Autodesk Inventor part; units mm, degrees
ref_plane "YZ Plane" through (0, 0, 0) normal (1, 0, 0) x (0, 1, 0)
ref_plane "XZ Plane" through (0, 0, 0) normal (0, 1, 0) x (-1, 0, 0)
ref_plane "XY Plane" through (0, 0, 0) normal (0, 0, 1) x (1, 0, 0)
sketch "Sketch1" plane through (0, 0, 0) normal (0, 0, 1) x (1, 0, 0)
  circle A0 centre (0, 0) radius 5
  circle A1 centre (0, 0) radius 7
  dimension "d0" = 10
  dimension "d1" = 14
extrude "Extrusion1" add sketch "Sketch1" along normal blind 12.7
sketch "Sketch2" plane through (0, 0, 12.7) normal (0, 0, 1) x (1, 0, 0)
  circle A0 centre (0, 0) radius 7
  dimension "d14" = 14
extrude "Extrusion2" add sketch "Sketch2" along normal blind 19.25
chamfer "Chamfer1" distance 0.4128 angle 45 1 edges at (-5, 0, 0)
thread "Thread1"
sketch "Sketch3" plane through (0, 0, 31.95) normal (0, 0, 1) x (1, 0, 0)
  circle A0 centre (0, 0) radius 5
  dimension "d11" = 10
extrude "Extrusion3" add sketch "Sketch3" along normal blind 12.7
thread "Thread2"
sketch "Sketch4" plane through (0, 0, 44.65) normal (0, 0, 1) x (1, 0, 0)
  line L0 (2.54, 0.635) -> (-2.54, 0.635)
  line L1 (-2.54, 0.635) -> (-2.54, -0.635)
  line L2 (-2.54, -0.635) -> (2.54, -0.635)
  line L3 (2.54, -0.635) -> (2.54, 0.635)
  line L4 (2.54, 0.635) -> (-2.54, -0.635) construction
  line L5 (-2.54, 0.635) -> (2.54, -0.635) construction
  point P0 (0, 0)
  dimension "d17" = 5.08
  dimension "d18" = 1.27
extrude "Extrusion4" cut sketch "Sketch4" against normal through all
properties part number "Pedal Shaft Extender Right"
Could you check a few things on this model? Use its own coordinates, in mm. A direction names the side the tool comes from. Round coordinates to 2 decimals unless told otherwise and drop trailing zeros. Write each loop counter-clockwise with the first axis right and the second up, starting at its lowest first coordinate (ties: lowest second). Pieces come first, ordered by that corner, then holes. Notation, with made-up numbers: M 86,56 L 145,56 A21 cw 145,79 Z; hole C 16,56.25 d3. An arc over 180 degrees is marked long. Answer in a Markdown table with one row per item. Add a question column.
Q1. Imagine slicing it at C-C (z = 10.5). Please give me the cut outline in (x, y), then the cut area to 3 significant figures.
Q2. If I drill on line 1 (Y direction, x = 0, z = 14) (3 decimals); line 2 (Z direction, x = 1.5, y = -6); line 3 (Y direction, x = -2.25, z = 22) (3 decimals), over which ranges is the centre line in solid material (lowest first)? Write a range as from..to.
Q3. If we mould it in two halves opening along Y, with no side actions, what happens to faces 1 (the cylindrical face through (-1.08, 4.88, 38.21)), 2 (the flat face through (0, -1, 44.65)), 3 (the flat face through (0, 0.635, 29))? For each: +Y half, -Y half, draft (parallel to the pull), parting line (faces both ways), or undercut.
Q4. Imagine slicing it at A-A (y = 0). Please give me the cut outline in (x, z).
Q5. Imagine slicing it at B-B (x = 0). Please give me the cut outline in (y, z) (3 decimals).
Q6. Will these pins go through, and if not, where does the flat tip stop? pin 1 Ø8 at (y, z) = (1, 39) entering from -X; pin 2 Ø1 at (x, z) = (-2, 35) entering from +Y; pin 3 Ø1 at (y, z) = (-4, 33.5) entering from -X.
Q7. On a 3-axis mill with a long thin cutter (end or side, diameter ignored), from which of +Z, -Z, +X, -X, +Y, -Y can I reach the whole of each face in a straight line? I mean faces 4 (the cylindrical face through (-1.08, 4.88, 6.47)), 5 (the flat face through (-2.54, 0, 29)), 6 (the flat face through (-2, 5, 31.95)), 7 (the flat face through (4, -4, 0)). Say none if no direction works.
Q8. Imagine slicing it at D-D (z = 42.5). Please give me the cut outline in (x, y) (3 decimals), then the cut area to 3 significant figures.
Values:
| question | item | result |
|---|---|---|
| 1 | outline | C 0,0 d14; hole C 0,0 d10 |
| 1 | area | 75.4 mm^2 |
| 2 | line 1 | -7..-0.635, 0.635..7 |
| 2 | line 2 | 0..31.95 |
| 2 | line 3 | -6.629..-0.635, 0.635..6.629 |
| 3 | face 1 | parting line |
| 3 | face 2 | draft |
| 3 | face 3 | undercut |
| 4 | outline | M -7,0 L -5.41,0 L -5,0.41 L -5,12.7 L -2.54,12.7 L -2.54,44.65 L -5,44.65 L -5,31.95 L -7,31.95 Z; M 2.54,12.7 L 5,12.7 L 5,0.41 L 5.41,0 L 7,0 L 7,31.95 L 5,31.95 L 5,44.65 L 2.54,44.65 Z |
| 5 | outline | M -7,0 L -5.413,0 L -5,0.413 L -5,12.7 L -0.635,12.7 L -0.635,44.65 L -5,44.65 L -5,31.95 L -7,31.95 Z; M 0.635,12.7 L 5,12.7 L 5,0.413 L 5.413,0 L 7,0 L 7,31.95 L 5,31.95 L 5,44.65 L 0.635,44.65 Z |
| 6 | pin 1 | x = -5 |
| 6 | pin 2 | y = 4.77 |
| 6 | pin 3 | x = -3.57 |
| 7 | face 4 | -Z |
| 7 | face 5 | +Z, -Z |
| 7 | face 6 | +Z |
| 7 | face 7 | -Z, +X, -X, +Y, -Y |
| 8 | outline | C 0,0 d10; hole M -2.54,-0.635 L 2.54,-0.635 L 2.54,0.635 L -2.54,0.635 Z |
| 8 | area | 72.1 mm^2 |
